from build123d import *

# Parameters (mm, degrees)
ESQUISSE1_W                  = 40
ESQUISSE1_H                  = 30
BOSS_EXTRU_1_DEPTH           = 5
ENL_V_MAT_EXTRU_1_DEPTH      = 51.249378106
ENL_V_MAT_EXTRU_1_DEPTH_BACK = 51.249378106
ESQUISSE2_R                  = 1.5
ESQUISSE2_R_2                = 2.5
CHANFREIN1_SIZE              = 10
CONG_1_R                     = 5


with BuildPart() as part:
    # Esquisse1 → Boss.-Extru.1 (new body)
    with BuildSketch(Plane.XY):
        with Locations((20, 15)):
            Rectangle(ESQUISSE1_W, ESQUISSE1_H)
    extrude(amount=BOSS_EXTRU_1_DEPTH)

    # Esquisse2 → Enlèv. mat.-Extru.1 (cut, two sides: drawn at the far end of the back side and taken through both)
    with BuildSketch(Plane.XY.offset(5).offset(-ENL_V_MAT_EXTRU_1_DEPTH_BACK)):
        with Locations((8, 23)):
            Circle(ESQUISSE2_R)
        with Locations(Location((32, 23, 0), (0, 0, 180))):
            Circle(ESQUISSE2_R)
        with Locations((20, 7)):
            Circle(ESQUISSE2_R_2)
    extrude(amount=ENL_V_MAT_EXTRU_1_DEPTH + ENL_V_MAT_EXTRU_1_DEPTH_BACK, mode=Mode.SUBTRACT)

    # Chanfrein1
    chanfrein1_edges = [part.edges().sort_by_distance(p)[0] for p in [
        (40, 0, 2.5),
        (0, 0, 2.5),
    ]]
    chamfer(chanfrein1_edges, length=CHANFREIN1_SIZE)

    # Congé1
    cong_1_edges = [part.edges().sort_by_distance(p)[0] for p in [
        (0, 30, 2.5),
        (40, 30, 2.5),
    ]]
    fillet(cong_1_edges, radius=CONG_1_R)


solid = part.part
The listing builds one solid part. Answer for the finished solid, in the listing's coordinates (mm). Round coordinates to 2 decimals unless told otherwise and drop trailing zeros. Order: outer loops, then holes, each group sorted by start corner. A loop starts at its lowest first (then second) coordinate and runs counter-clockwise, first axis right, second up. Notation, with made-up numbers: (80, -12) -> (96, -12) arc R21 cw to (96, 8) -> close; hole circle Ø4 at (17.5, -30). An arc over 180 degrees is marked (long way). Write each question's results on one line, items separated by ' | '. Start each with the question number.
Q1. Find section C-C (z = 3.4). Determine the outline of the cut face in (x, y).
Q2. Find section B-B (x = 20). Determine the outline of the cut face in (y, z), then the cut area to 3 significant figures.
Q3. Straight lines are drawn through the part: probe 1 along Y at (x, z) = (20, 2.85); probe 2 along X at (y, z) = (24.25, 3.4); probe 3 along Y at (x, z) = (32, 2.8). For each, find the intervals that lie inside material, in ascending order. Write a range as from..to.
Q4. Find section D-D (y = 23). Determine the outline of the cut face in (x, z).
Q5. This flat-tipped pin is pushed along its axis until it touches: pin 1 (4 mm diameter, centred on x = 8, y = 23, fed in from -Z). Where does it stop, or does it pass through?
Q6. Find section A-A (y = 7). Determine the outline of the cut face in (x, z), then the cut area to 3 significant figures.
Q7. The mould has two halves that part along X. Classify faces 1 (the cylindrical face through (33.11, 21.99, 2.46)), 2 (the flat face through (20, 15, 0)), 3 (the cylindrical face through (1, 28, 3)): pulls with the +X half, pulls with the -X half, needs draft (parallel to the pull), parting line crosses it, or undercut.
Worked answers:
1) outline: (0, 10) -> (10, 0) -> (30, 0) -> (40, 10) -> (40, 25) arc R5 ccw to (35, 30) -> (5, 30) arc R5 ccw to (0, 25) -> close; hole circle Ø3 at (8, 23); hole circle Ø5 at (20, 7); hole circle Ø3 at (32, 23)
2) outline: (0, 0) -> (4.5, 0) -> (4.5, 5) -> (0, 5) -> close; (9.5, 0) -> (30, 0) -> (30, 5) -> (9.5, 5) -> close | area: 125 mm2
3) probe 1: y = 0..4.5, 9.5..30 | probe 2: x = 0..7.17, 8.83..31.17, 32.83..40 | probe 3: y = 2..21.5, 24.5..30
4) outline: (0, 0) -> (6.5, 0) -> (6.5, 5) -> (0, 5) -> close; (9.5, 0) -> (30.5, 0) -> (30.5, 5) -> (9.5, 5) -> close; (33.5, 0) -> (40, 0) -> (40, 5) -> (33.5, 5) -> close
5) pin 1: stops at z = 0
6) outline: (3, 0) -> (17.5, 0) -> (17.5, 5) -> (3, 5) -> close; (22.5, 0) -> (37, 0) -> (37, 5) -> (22.5, 5) -> close | area: 145 mm2
7) face 1: undercut | face 2: needs draft | face 3: pulls with the -X half
